Part print with two shaded views. Sizes in mm from the minimum x, y, z corner. Give positions to 0.01 mm unless a question says otherwise; leave off trailing zeros. Write each loop counter-clockwise with the first axis right and the second up, starting at its lowest first coordinate (ties: lowest second). Pieces come first, ordered by that corner, then holes. Notation, with made-up numbers: (-33.75, 26.5) -> (2.25, 26.5) arc R24 cw to (2.25, 65.5) -> close; hole circle Ø9 at (22.5, 65). An arc over 180 degrees is marked (long way). Use one line per item in the form item = value. Start each with the question number.
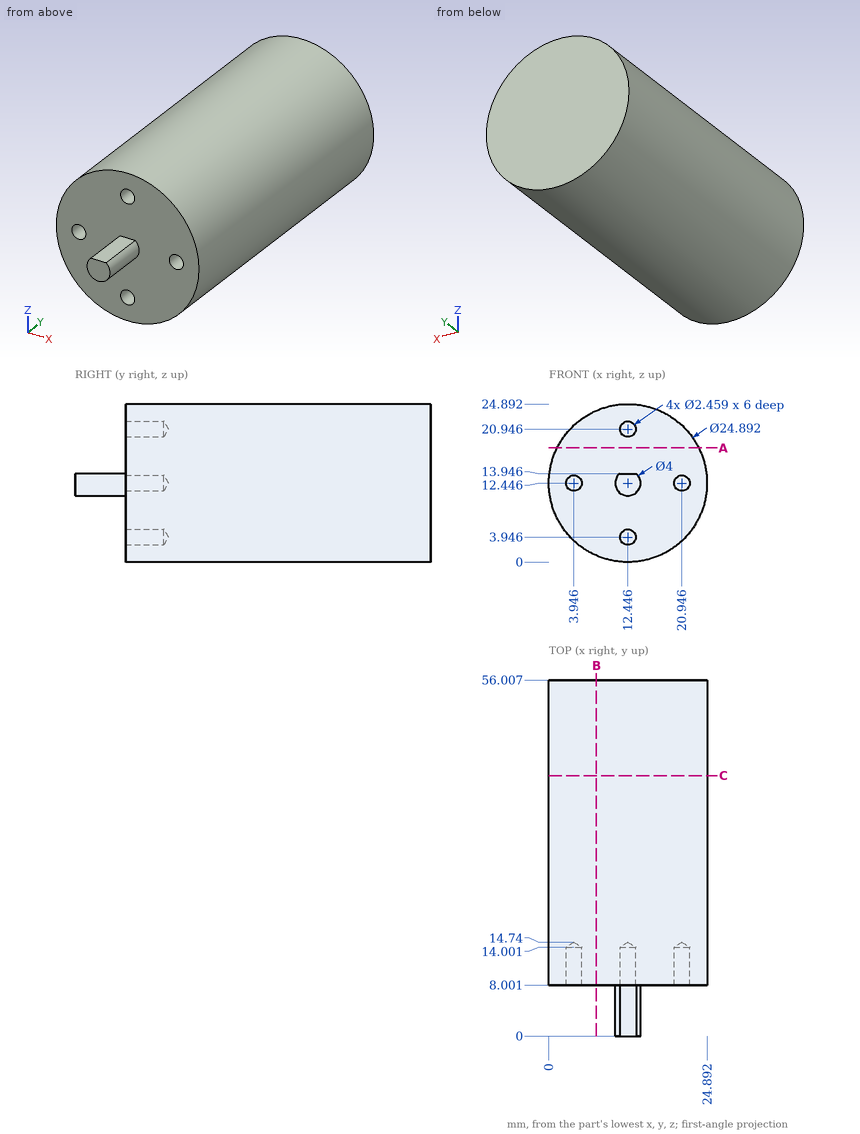
1) Pin check, flat tips, straight feed: pin 1 (1.5 mm diameter, centred on x = 10.5, y = 39.5, fed in from +Z); pin 2 (12.5 mm diameter, centred on x = 7, z = 16, fed in from -Y); pin 3 (3 mm diameter, centred on y = 42.5, z = 4, fed in from +X); pin 4 (2 mm diameter, centred on x = 12.5, y = 5.5, fed in from +Z). Stop position of each tip, or through.
2) Cut at B-B (x = 7.5). Give the cut face in (y, z) (1 decimal), and give its area (3 significant figures).
3) Cut at C-C (y = 41). Give the cut face in (x, z), and give its area (3 significant figures).
4) Cut at A-A (z = 18). Give the cut face in (x, y), and give its area (3 significant figures).
5) Wall check: line 1 along Y through (x, z) = (11.25, 16); line 2 along X through (y, z) = (50.5, 14.25); line 3 along X through (y, z) = (38, 16). Give the ranges that are in metal, low to high. Write a range as from..to.
Final values:
q1.pin_1 = 24.83
q1.pin_2 = 0
q1.pin_3 = 22.77
q1.pin_4 = 13.95
q2.outline = (8, 1) -> (56, 1) -> (56, 23.9) -> (8, 23.9) -> close
q2.area = 1,100 mm^2
q3.outline = circle Ø24.89 at (12.45, 12.45)
q3.area = 487 mm^2
q4.outline = (1.31, 8) -> (23.58, 8) -> (23.58, 56.01) -> (1.31, 56.01) -> close
q4.area = 1,070 mm^2
q5.line_1 = 8..56.01
q5.line_2 = 0.13..24.76
q5.line_3 = 0.52..24.37
